Answer from the drawing. Dimensions are ordinates in mm from the lowest x, y and z of the part. Round coordinates to 2 decimals unless told otherwise and drop trailing zeros. Write each loop counter-clockwise with the first axis right and the second up, starting at its lowest first coordinate (ties: lowest second). Pieces come first, ordered by that corner, then holes. Notation, with made-up numbers: M -1.5,72 L 35.5,72 A19 cw 35.5,84 Z; hole C 56,77.5 d3. An arc over 180 degrees is marked long. Answer as CSV lines item,"result". Start each with the question number.
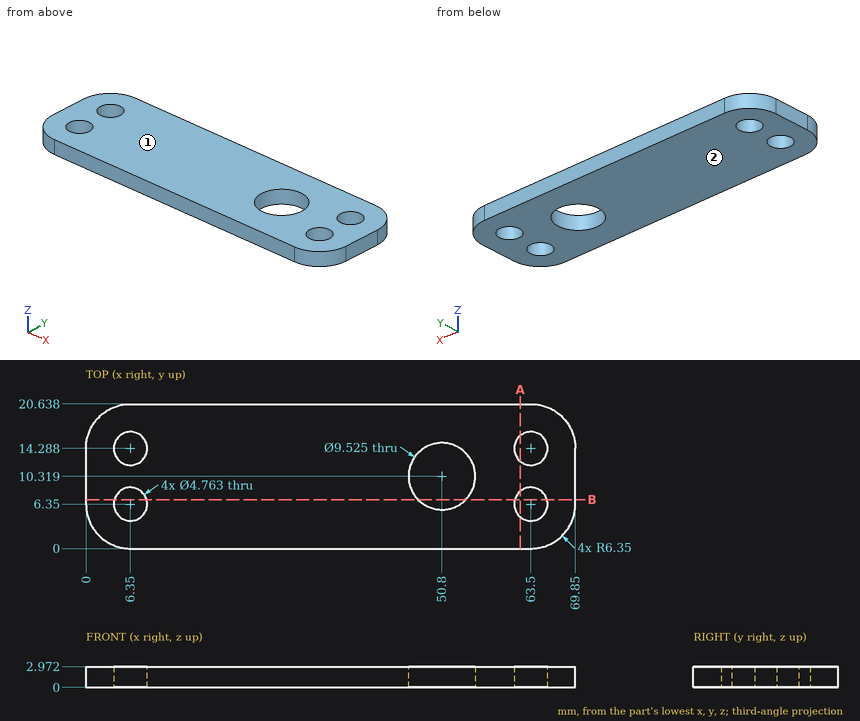
Q1. This flat-tipped pin is pushed along its axis until it touches: P1, Ø4, axis at x = 6.35, y = 14.29, coming from the -Z side. Where does it stop, or does it pass through?
Q2. Find section A-A (x = 62). Determine the outline of the cut face in (y, z).
Q3. Straight lines are drawn through the part: L1, parallel to Y at x = 63.5, z = 0.95; L2, parallel to X at y = 10.25, z = 0.4; L3, parallel to X at y = 16, z = 0.55 (1 decimal). For each, find the intervals that lie inside material, in ascending order.
Q4. The mould has two halves that part along Z. Classify the marked faces 1 and 2: +Z half, -Z half, draft (parallel to the pull), parting line (faces both ways), or undercut.
Q5. Find section B-B (y = 7). Count the separate pieces of the cut face and the enclosed holes in it, plus the area to 3 significant figures.
Reported:
1,P1,"passes through"
2,outline,"M 0,0 L 4.5,0 L 4.5,2.97 L 0,2.97 Z; M 8.2,0 L 12.44,0 L 12.44,2.97 L 8.2,2.97 Z; M 16.14,0 L 20.64,0 L 20.64,2.97 L 16.14,2.97 Z"
3,L1,"y = 0 to 3.97, 8.73 to 11.91, 16.67 to 20.64"
3,L2,"x = 0 to 46.04, 55.56 to 69.85"
3,L3,"x = 0.2 to 4.7, 8 to 61.8, 65.2 to 69.6"
4,face 1,"+Z half"
4,face 2,"-Z half"
5,separate pieces,"4"
5,enclosed holes,"0"
5,area,"160 mm2"
